Geometry check sheet. Reference: the model listing, model coordinates, mm. Face numbers are marked on the shaded views. Give positions to 0.01 mm unless a question says otherwise; leave off trailing zeros. Write each loop counter-clockwise with the first axis right and the second up, starting at its lowest first coordinate (ties: lowest second). Pieces come first, ordered by that corner, then holes. Notation, with made-up numbers: M -33,53 L -16,53 A20 ccw -16,86 Z; hole C 36.5,23 d7. An arc over 180 degrees is marked long. One line per item, written item: value. Start each with the question number.
1. Gauge pin test, flat ends, axial feed: pin 1 (1 mm diameter, centred on x = 29.5, y = -7.5, fed in from -Z); pin 2 (8 mm diameter, centred on x = 4, y = -6.5, fed in from +Z); pin 3 (5 mm diameter, centred on x = 60.21, y = -55.15, fed in from +Z). Record the tip position at first contact, or that the pin passes through.
2. Cross-section at A-A on z = 3.5. Record the cut outline in (x, y).
3. Cross-section at B-B on y = 37.5. Record the cut outline in (x, z), then the cut area to 3 significant figures.
4. Cross-section at C-C on x = 56. Record the cut outline in (y, z), then the cut area to 3 significant figures.
5. Scan lines: line 1 (X direction, y = 16, z = 4.5); line 2 (Y direction, x = 39, z = 11); line 3 (Z direction, x = -58.5, y = -4.5). Record each from-to range of solid material in increasing order.
6. Release check for a two-part mould opening along Y. For the marked faces 1, 2, 3 and 4 record: pulls with the +Y half, pulls with the -Y half, needs draft (parallel to the pull), parting line crosses it, or undercut.
Autodesk Inventor part; units mm, degrees
ref_plane "YZ Plane" through (0, 0, 0) normal (1, 0, 0) x (0, 1, 0)
ref_plane "XZ Plane" through (0, 0, 0) normal (0, 1, 0) x (-1, 0, 0)
ref_plane "XY Plane" through (0, 0, 0) normal (0, 0, 1) x (1, 0, 0)
sketch "스케치1" plane through (0, 0, 0) normal (0, 0, 1) x (1, 0, 0)
  line L0 (65, -60) -> (-65, -60)
  line L1 (-65, -60) -> (-65, 60)
  line L2 (-65, 60) -> (65, 60)
  line L3 (65, 60) -> (65, -60)
  line L4 (65, -60) -> (-65, 60) construction
  line L5 (-65, -60) -> (65, 60) construction
  line L6 (63, 58) -> (-63, 58) construction
  line L7 (-63, 58) -> (-63, -58) construction
  line L8 (-63, -58) -> (63, -58) construction
  line L9 (63, -58) -> (63, 58) construction
  point P0 (0, 0)
  dimension "d0" = 130
  dimension "d1" = 120
  dimension "d2" = 2
extrude "돌출1" add sketch "스케치1" along normal blind 12
shell "쉘1" thickness 1.2 removed faces 1 at (21.6667, 20, 12)
sketch "스케치2" plane through (-63.8, -58.8, 1.2) normal (0, 0, 1) x (1, 0, 0)
  point P0 (63.8, 58.8)
sketch "스케치3" plane through (-63.8, -58.8, 1.2) normal (0, 0, 1) x (1, 0, 0)
  circle A0 centre (92.0039, 113.6118) radius 2.7
  circle A1 centre (4.0037, 3.6486) radius 2.7
  circle A2 centre (4.0037, 113.6118) radius 2.7
  circle A3 centre (124.0062, 3.6486) radius 2.7
  point P0 (63.8, 58.8)
  dimension "d6" = 5.4
  dimension "d7" = 5.4
  dimension "d8" = 5.4
  dimension "d9" = 5.4
extrude "돌출2" cut sketch "스케치3" against normal blind 12
properties part number "240621_pt1"
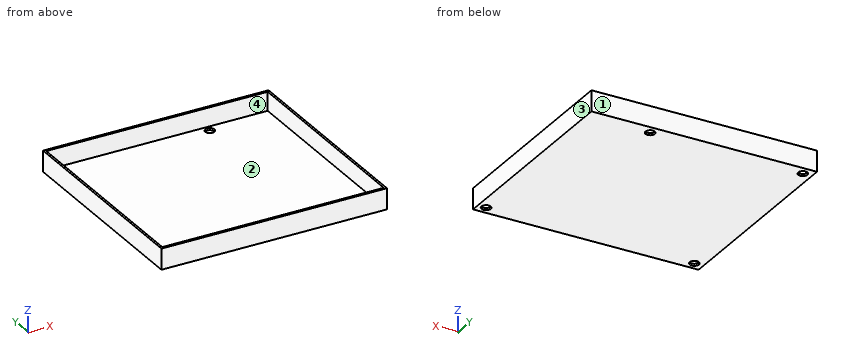
Report:
1. pin 1: stops at z = 0
1. pin 2: stops at z = 1.2
1. pin 3: passes through
2. outline: M -65,-60 L 65,-60 L 65,60 L -65,60 Z; hole M -63.8,-58.8 L 63.8,-58.8 L 63.8,58.8 L -63.8,58.8 Z
3. outline: M -65,0 L 65,0 L 65,12 L 63.8,12 L 63.8,1.2 L -63.8,1.2 L -63.8,12 L -65,12 Z
3. area: 182 mm^2
4. outline: M -60,0 L 60,0 L 60,12 L 58.8,12 L 58.8,1.2 L -58.8,1.2 L -58.8,12 L -60,12 Z
4. area: 170 mm^2
5. line 1: x = -65 to -63.8, 63.8 to 65
5. line 2: y = -60 to -58.8, 58.8 to 60
5. line 3: z = 0 to 1.2
6. face 1: pulls with the +Y half
6. face 2: undercut
6. face 3: needs draft
6. face 4: undercut
